Can you work these out from the model? Positions are in its coordinate system, mm. A direction names the side the tool comes from. Round coordinates to 2 decimals unless told otherwise and drop trailing zeros. Loops run counter-clockwise (first coordinate to the right, second up) from the corner with the lowest first, then second, coordinate; pieces in that order, holes last.
from build123d import *

# Parameters (mm, degrees)
SKETCH_1_R          = 4.5
SKETCH_1_R_2        = 4
EXTRUDE_1_DEPTH     = 3.5
SKETCH_1_3_R        = 5.5
SKETCH_1_3_R_2      = 4.5
EXTRUDE_2_DEPTH     = 3
SKETCH_1_4_R        = 6
SKETCH_1_4_R_2      = 5.5
EXTRUDE_3_DEPTH     = 3.5
SKETCH_1_5_R        = 5.5
SKETCH_1_5_R_2      = 4.5
CUT_EXTRUDE_1_DEPTH = 0.5


with BuildPart() as part:
    # Sketch 1 → Extrude 1 (new body)
    with BuildSketch(Plane(origin=(0, 0, 0), x_dir=(1, 0, 0), z_dir=(0, 1, 0))):
        with Locations(Location((0, 0, 0), (0, 0, 270))):
            Circle(SKETCH_1_R)
        with Locations(Location((0, 0, 0), (0, 0, 270))):
            Circle(SKETCH_1_R_2, mode=Mode.SUBTRACT)
    extrude(amount=EXTRUDE_1_DEPTH)

    # Sketch 1_3 → Extrude 2 (add)
    with BuildSketch(Plane(origin=(0, 0, 0), x_dir=(1, 0, 0), z_dir=(0, 1, 0))):
        with Locations(Location((0, 0, 0), (0, 0, 270))):
            Circle(SKETCH_1_3_R)
        with Locations(Location((0, 0, 0), (0, 0, 270))):
            Circle(SKETCH_1_3_R_2, mode=Mode.SUBTRACT)
    extrude(amount=EXTRUDE_2_DEPTH)

    # Sketch 1_4 → Extrude 3 (add)
    with BuildSketch(Plane(origin=(0, 0, 0), x_dir=(1, 0, 0), z_dir=(0, 1, 0))):
        with Locations(Location((0, 0, 0), (0, 0, 270))):
            Circle(SKETCH_1_4_R)
        with Locations(Location((0, 0, 0), (0, 0, 270))):
            Circle(SKETCH_1_4_R_2, mode=Mode.SUBTRACT)
    extrude(amount=EXTRUDE_3_DEPTH)

    # Sketch 1_5 → Cut-Extrude 1 (cut)
    with BuildSketch(Plane(origin=(0, 0, 0), x_dir=(1, 0, 0), z_dir=(0, 1, 0))):
        with Locations(Location((0, 0, 0), (0, 0, 270))):
            Circle(SKETCH_1_5_R)
        with Locations(Location((0, 0, 0), (0, 0, 270))):
            Circle(SKETCH_1_5_R_2, mode=Mode.SUBTRACT)
    extrude(amount=CUT_EXTRUDE_1_DEPTH, mode=Mode.SUBTRACT)


solid = part.part
(1) If we section it at A-A, the plane y = 3.25: List the corners of the cut face in (x, z) for me.
Worked answers:
outline: circle Ø12 at (0, 0); circle Ø9 at (0, 0); hole circle Ø11 at (0, 0); hole circle Ø8 at (0, 0)
(2) Will these pins go through, and if not, where does the flat tip stop? P1, Ø2, axis at x = -3, y = 1, coming from the -Z side; P2, Ø1, axis at y = 2, z = 3.5, coming from the -X side.
Worked answers:
P1: stops at z = -5.66
P2: stops at x = -5.2
(3) If we section it at C-C, the plane z = 0: List the corners of the cut face in (x, y) for me.
Worked answers:
outline: (-6, 0) - (-5.5, 0) - (-5.5, 0.5) - (-4.5, 0.5) - (-4.5, 0) - (-4, 0) - (-4, 3.5) - (-4.5, 3.5) - (-4.5, 3) - (-5.5, 3) - (-5.5, 3.5) - (-6, 3.5) - close; (4, 0) - (4.5, 0) - (4.5, 0.5) - (5.5, 0.5) - (5.5, 0) - (6, 0) - (6, 3.5) - (5.5, 3.5) - (5.5, 3) - (4.5, 3) - (4.5, 3.5) - (4, 3.5) - close
(4) If we section it at D-D, the plane y = 0.9: List the corners of the cut face in (x, z) for me.
Worked answers:
outline: circle Ø12 at (0, 0); hole circle Ø8 at (0, 0)
(5) For faces 1 (the flat face through (-3, 3.5, -3)), 2 (the flat face through (0, 3, -5)), 3 (the cylindrical face through (-5.37, 0.25, -1.19)), which set-ups out of +Z, -Z, +X, -X, +Y, -Y let a thin tool reach every point of the face, with its end or its side?
Worked answers:
face 1: +Z, -Z, +X, -X, +Y
face 2: +Y
face 3: -Y
(6) If I drill on line 1 (X direction, y = 3.25, z = 0); line 2 (Y direction, x = -4.75, z = -2.5); line 3 (X direction, y = 1.5, z = 3.5), over which ranges is the centre line in solid material (lowest first)?
Worked answers:
line 1: x = -6 to -5.5, -4.5 to -4, 4 to 4.5, 5.5 to 6
line 2: y = 0.5 to 3
line 3: x = -4.87 to -1.94, 1.94 to 4.87
(7) If we mould it in two halves opening along Z, with no side actions, what happens to faces 4 (the flat face through (-3, 0, -3)), 5 (the cylindrical face through (1.802, 1.726, 5.723)), 6 (the cylindrical face through (1.352, 3.246, 4.292))? For each: released by +Z, released by -Z, zero draft, split by the parting line, or undercut.
Worked answers:
face 4: zero draft
face 5: split by the parting line
face 6: undercut
(8) If we section it at B-B, the plane x = 0: List the corners of the cut face in (y, z) for me, then the cut area to 3 significant figures.
Worked answers:
outline: (0, -6) - (3.5, -6) - (3.5, -5.5) - (3, -5.5) - (3, -4.5) - (3.5, -4.5) - (3.5, -4) - (0, -4) - (0, -4.5) - (0.5, -4.5) - (0.5, -5.5) - (0, -5.5) - close; (0, 4) - (3.5, 4) - (3.5, 4.5) - (3, 4.5) - (3, 5.5) - (3.5, 5.5) - (3.5, 6) - (0, 6) - (0, 5.5) - (0.5, 5.5) - (0.5, 4.5) - (0, 4.5) - close
area: 12.0 mm2
